Model file for the job. Use its own axes, mm. Give positions to 0.01 mm unless a question says otherwise; leave off trailing zeros. Write each loop counter-clockwise with the first axis right and the second up, starting at its lowest first coordinate (ties: lowest second). Pieces come first, ordered by that corner, then holes.
Autodesk Inventor part; units mm, degrees
ref_plane "YZ Plane" through (0, 0, 0) normal (1, 0, 0) x (0, 1, 0)
ref_plane "XZ Plane" through (0, 0, 0) normal (0, 1, 0) x (-1, 0, 0)
ref_plane "XY Plane" through (0, 0, 0) normal (0, 0, 1) x (1, 0, 0)
sketch "Sketch1" plane through (0, 0, 0) normal (0, 0, 1) x (1, 0, 0)
  circle A0 centre (0, 0) radius 11
  dimension "d0" = 22
extrude "Extrusion1" add sketch "Sketch1" along normal blind 1
sketch "Sketch2" plane through (0, 0, 1) normal (0, 0, 1) x (1, 0, 0)
  circle A0 centre (0, 0) radius 11
  point P0 (9.64, 0)
  dimension "d3" = 9.64
hole "Hole1" at (9.64, 0, 1) direction (0, 0, -1) diameter 1.181 depth 8
pattern_circular "Circular Pattern1" count 3 over 360 about axis through (0, 0, -10) along (0, 0, 1) of "Hole1"
properties part number "Electronics"
1. Slice it at C-C, the plane x = 9.64. Write the cut outline in (y, z), and give its area (3 significant figures).
Calculated:
outline: (-5.3, 0) - (-0.59, 0) - (-0.59, 1) - (-5.3, 1) - close; (0.59, 0) - (5.3, 0) - (5.3, 1) - (0.59, 1) - close
area: 9.42 mm2
2. Probe probe 1 along Y at (x, z) = (-5, 0.75); probe 2 along X at (y, z) = (8, 0.2); probe 3 along X at (y, z) = (8.75, 0.45). List the from-to ranges inside material, lowest first.
Calculated:
probe 1: y = -9.8 to -8.91, -7.79 to 7.79, 8.91 to 9.8
probe 2: x = -7.55 to -5.3, -4.34 to 7.55
probe 3: x = -6.67 to -5.25, -4.39 to 6.67
3. Pin check, flat tip, straight feed: P1, Ø1.1, axis at x = -4.82, y = -8.35, coming from the +Z side. Stop position of the tip, or through.
Calculated:
P1: passes through
4. Slice it at A-A, the plane y = 0. Write the cut outline in (x, z).
Calculated:
outline: (-11, 0) - (9.05, 0) - (9.05, 1) - (-11, 1) - close; (10.23, 0) - (11, 0) - (11, 1) - (10.23, 1) - close
5. Slice it at B-B, the plane x = -4.82. Write the cut outline in (y, z).
Calculated:
outline: (-9.89, 0) - (-8.94, 0) - (-8.94, 1) - (-9.89, 1) - close; (-7.76, 0) - (7.76, 0) - (7.76, 1) - (-7.76, 1) - close; (8.94, 0) - (9.89, 0) - (9.89, 1) - (8.94, 1) - close
6. Slice it at D-D, the plane z = 0.2. Write the cut outline in (x, y), and give its area (3 significant figures).
Calculated:
outline: circle Ø22 at (0, 0); hole circle Ø1.18 at (-4.82, -8.35); hole circle Ø1.18 at (-4.82, 8.35); hole circle Ø1.18 at (9.64, 0)
area: 377 mm2
